Part model, mm, in its own coordinate system. A direction names the side the tool comes from. Round coordinates to 2 decimals unless told otherwise and drop trailing zeros. Loops run counter-clockwise (first coordinate to the right, second up) from the corner with the lowest first, then second, coordinate; pieces in that order, holes last. Notation, with made-up numbers: (0, 57) -> (22, 57) arc R29 ccw to (22, 79) -> close; hole circle Ø9 at (17.5, 56.25). An arc over 180 degrees is marked (long way). Use a Markdown table: item, result. Add a question column.
Item 1: Probe line 1 (Z direction, x = -0.5, y = 7); line 2 (X direction, y = 58, z = 0); line 3 (Z direction, x = 8, y = 45.5). List the from-to ranges inside material, lowest first. Write a range as [from, to].
Item 2: Which spindle directions (+Z, -Z, +X, -X, +Y, -Y) get a long thin tool onto all of the face, cutting with end or side? Do faces 4 (the face through (-5.453, 4.86, 0.716)), 5 (the face through (-7.04, 8.34, 0.92)). Say none if no direction does.
Item 3: Two-plate mould, pull along X, no slides. Class faces 1 (the face through (-13.97, 58.9, -44.35)), 2 (the face through (31, 62, -31)), 3 (the face through (-36.679, 59.03, -23.385)): pulls with the +X half, pulls with the -X half, needs draft (parallel to the pull), parting line crosses it, or undercut.
Item 4: Flat gauge pins, fed straight in: pin 1 (6 mm diameter, centred on x = 13, z = 16, fed in from +Y); pin 2 (3 mm diameter, centred on x = -9.5, z = 32, fed in from +Y); pin 3 (10 mm diameter, centred on x = 25.5, y = 50, fed in from -Z); pin 4 (19.5 mm diameter, centred on x = -0.5, z = 3, fed in from -Y). Where does each tip first touch, or does it go through?
Item 5: Cut at A-A, the plane y = 26. List the corners of the cut face in (x, z).
```python
from build123d import *

# Parameters (mm, degrees)
FILLET1_R      = 10
CHAMFER1_SIZE  = 0.4
CHAMFER1_SIZE2 = 4.572020921


with BuildPart() as part:
    # Sketch1 → Revolve1 (revolve)
    with BuildSketch(Plane.XY, mode=Mode.PRIVATE) as revolve1_sk:
        Polygon((5.5, 0), (7.1, 0), (7.1, 12), (12.1, 12), (46.5, 52), (46.5, 62), (43.5, 62), (43.5, 52), (5.5, 14), align=None)
    revolve(revolve1_sk.sketch.rotate(Axis((0, 0, 0), (0, 1, 0)), 90), axis=Axis((0, 0, 0), (0, 1, 0)))

    # Fillet1
    fillet1_edges = [part.edges().sort_by_distance(p)[0] for p in [
        (0, 14, 5.5),
        (0, 52, 43.5),
        (0, 52, 46.5),
    ]]
    fillet(fillet1_edges, radius=FILLET1_R)

    # Chamfer1
    chamfer1_edges = [part.edges().sort_by_distance(p)[0] for p in [
        (0, 0, 7.1),
    ]]
    chamfer1_side = [part.faces().sort_by_distance(p)[0] for p in [
        (0, 0, 5.700818326),
    ]]
    chamfer(chamfer1_edges, length=CHAMFER1_SIZE, length2=CHAMFER1_SIZE2, reference=chamfer1_side[0])


solid = part.part
```
A:
| question | item | result |
|---|---|---|
| 1 | line 1 | z = [-7.08, -5.48], [5.48, 7.08] |
| 1 | line 2 | x = [-46.5, -43.5], [43.5, 46.5] |
| 1 | line 3 | z = [-40.12, -36.12], [36.12, 40.12] |
| 2 | face 4 | +Y, -Y |
| 2 | face 5 | -Y |
| 3 | face 1 | parting line crosses it |
| 3 | face 2 | needs draft |
| 3 | face 3 | undercut |
| 4 | pin 1 | stops at y = 32.12 |
| 4 | pin 2 | stops at y = 43.38 |
| 4 | pin 3 | stops at z = -40.82 |
| 4 | pin 4 | stops at y = 0 |
| 5 | outline | circle Ø48.28 at (0, 0); hole circle Ø35 at (0, 0) |
